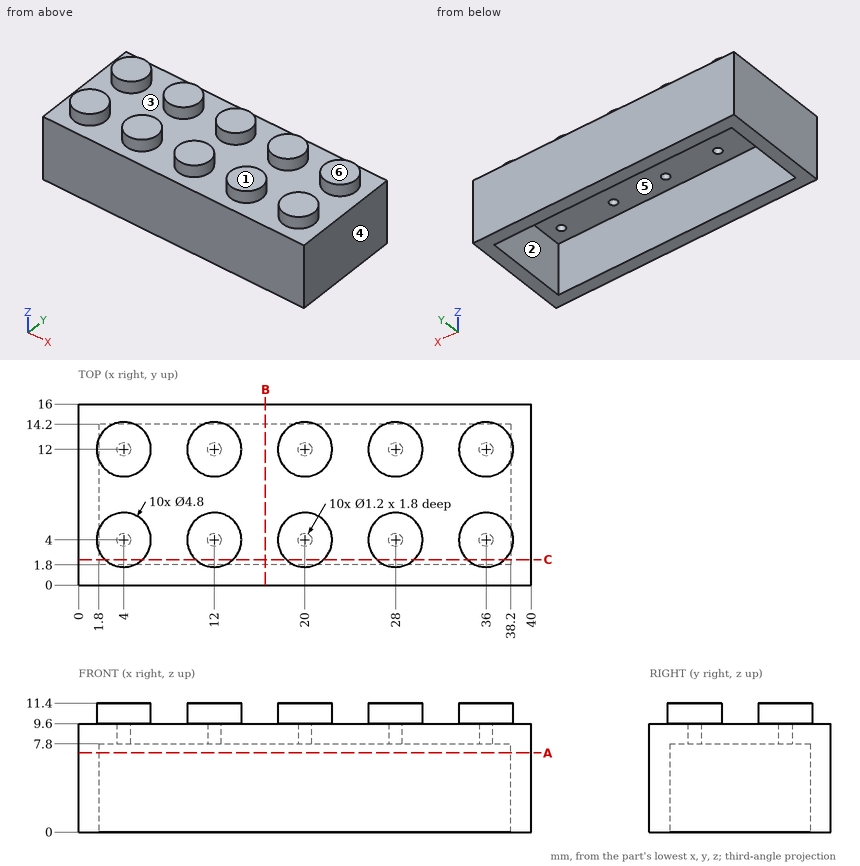
Verification items for this drawing (mm, ordinates from the low corner). A direction names the side the tool comes from. Give positions to 0.01 mm unless a question says otherwise; leave off trailing zeros. Order: outer loops, then holes, each group sorted by start corner. A loop starts at its lowest first (then second) coordinate and runs counter-clockwise, first axis right, second up.
1) Cross-section at A-A (z = 7). Record the boundary of the cut face in (x, y).
Results are:
outline: (0, 0) - (40, 0) - (40, 16) - (0, 16) - close; hole (1.8, 1.8) - (38.2, 1.8) - (38.2, 14.2) - (1.8, 14.2) - close
2) Draft check along X on the marked faces 4, 5 and 6. Enter one of: released by +X, released by -X, zero draft, split by the parting line, or undercut.
Results are:
face 4: released by +X
face 5: undercut
face 6: zero draft
3) Gauge pin test, flat ends, axial feed: pin 1 (0.6 mm diameter, centred on x = 4, y = 12, fed in from -Z); pin 2 (1.3 mm diameter, centred on x = 4, y = 4.5, fed in from -Z). Record the tip position at first contact, or that the pin passes through.
Results are:
pin 1: stops at z = 9.6
pin 2: stops at z = 7.8
4) Cross-section at C-C (y = 2.25). Record the boundary of the cut face in (x, z), then the cut area to 3 significant figures.
Results are:
outline: (0, 0) - (1.8, 0) - (1.8, 7.8) - (38.2, 7.8) - (38.2, 0) - (40, 0) - (40, 9.6) - (37.64, 9.6) - (37.64, 11.4) - (34.36, 11.4) - (34.36, 9.6) - (29.64, 9.6) - (29.64, 11.4) - (26.36, 11.4) - (26.36, 9.6) - (21.64, 9.6) - (21.64, 11.4) - (18.36, 11.4) - (18.36, 9.6) - (13.64, 9.6) - (13.64, 11.4) - (10.36, 11.4) - (10.36, 9.6) - (5.64, 9.6) - (5.64, 11.4) - (2.36, 11.4) - (2.36, 9.6) - (0, 9.6) - close
area: 130 mm2
5) Material ranges on probe 1 along X at (y, z) = (4, 8.5); probe 2 along Y at (x, z) = (26, 4.25); probe 3 along X at (y, z) = (4.25, 7), recorded low to high.
Results are:
probe 1: x = 0 to 3.4, 4.6 to 11.4, 12.6 to 19.4, 20.6 to 27.4, 28.6 to 35.4, 36.6 to 40
probe 2: y = 0 to 1.8, 14.2 to 16
probe 3: x = 0 to 1.8, 38.2 to 40
6) Cross-section at B-B (x = 16.5). Record the boundary of the cut face in (y, z).
Results are:
outline: (0, 0) - (1.8, 0) - (1.8, 7.8) - (14.2, 7.8) - (14.2, 0) - (16, 0) - (16, 9.6) - (0, 9.6) - close
7) Tool access check on the marked faces 1, 2 and 3. Record the directions out of +Z, -Z, +X, -X, +Y, -Y that give a thin tool (end or side, any length) a straight path to the whole face; none if there is none.
Results are:
face 1: +Z, +X, -X, +Y, -Y
face 2: -Z
face 3: +Z
